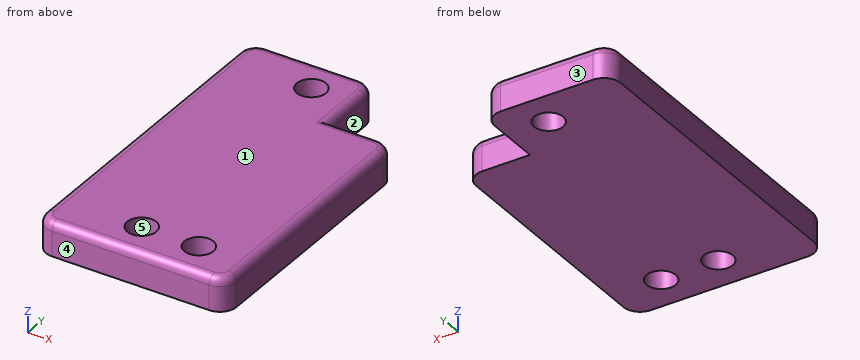
Autodesk Inventor part; units mm, degrees
ref_plane "Work Plane1" through (-7.86, -16.002, 12.7) normal (0, 0, 1) x (1, 0, 0)
ref_plane "YZ Plane" through (0, 0, 0) normal (1, 0, 0) x (0, 1, 0)
ref_plane "XZ Plane" through (0, 0, 0) normal (0, 1, 0) x (-1, 0, 0)
ref_plane "Work Plane1" through (-7.86, -16.002, 12.7) normal (0, 0, 1) x (1, 0, 0)
sketch "Sketch5" plane through (0, 0, 0) normal (0, 0, 1) x (1, 0, 0)
  line L0 (7.248, 20) -> (7.248, 11.68)
  line L1 (-5.86, 20) -> (7.248, 20)
  arc A0 (-5.86, 20) -> (-7.86, 18) centre (-5.86, 18) ccw
  line L2 (-7.86, 11.68) -> (-7.86, 18)
  line L3 (-3.792, 11.68) -> (-7.86, 11.68)
  line L4 (-3.792, 16.252) -> (-3.792, 11.68)
  line L5 (-0.752, 16.252) -> (-3.792, 16.252)
  line L6 (-0.752, 11.68) -> (-0.752, 16.252)
  line L7 (7.248, 11.68) -> (-0.752, 11.68)
  arc A1 (-7.86, -18) -> (-5.86, -20) centre (-5.86, -18) ccw
  line L8 (13, -20) -> (-5.86, -20)
  arc A2 (13, -20) -> (15, -18) centre (13, -18) ccw
  line L9 (15, -11.68) -> (15, -18)
  line L10 (-0.752, -11.68) -> (15, -11.68)
  line L11 (-0.752, -16.252) -> (-0.752, -11.68)
  line L12 (-3.792, -16.252) -> (-0.752, -16.252)
  line L13 (-3.792, -11.68) -> (-3.792, -16.252)
  line L14 (-7.86, -11.68) -> (-3.792, -11.68)
  line L15 (-7.86, -18) -> (-7.86, -11.68)
  line L16 (-0.752, 16.252) -> (-3.792, 16.252)
  line L17 (-3.792, 16.252) -> (-3.792, -16.252)
  line L18 (-3.792, -16.252) -> (-0.752, -16.252)
  line L19 (-0.752, -16.252) -> (-0.752, 16.252)
  line L20 (7.248, 11.68) -> (-7.86, 11.68)
  line L21 (-7.86, 11.68) -> (-7.86, -11.68)
  line L22 (-7.86, -11.68) -> (7.248, -11.68)
  line L23 (7.248, -11.68) -> (7.248, 11.68)
  line L24 (15, 11.43) -> (-1.002, 11.43)
  line L25 (15, 11.43) -> (7.248, 11.43)
  line L26 (7.248, 11.43) -> (7.248, -11.68)
  line L27 (7.248, -11.68) -> (15, -11.68)
  line L28 (15, -11.68) -> (15, 11.43)
  point P0 (0, 0)
extrude "Extrusion3" add sketch "Sketch5" along normal blind 4
sketch "Sketch6" plane through (0, 0, 4) normal (0, 0, 1) x (1, 0, 0)
  line L0 (7.248, 11.43) -> (7.248, 20)
  line L1 (7.248, 15.715) -> (2.248, 15.715)
  circle A0 centre (2.248, 15.715) radius 1.75
  line L2 (14.9228, 0) -> (0, 0)
  line L3 (7.248, 20) -> (7.248, 15.715)
  line L4 (15, -18) -> (15, 11.43)
  line L5 (15, -20) -> (15, -15.715)
  line L6 (15, -15.715) -> (-7.86, -15.715)
  line L7 (-7.86, 18) -> (-7.86, -18)
  line L8 (15, -15.715) -> (9, -15.715)
  circle A1 centre (9, -15.715) radius 1.75
  line L9 (-7.86, -15.715) -> (2.14, -15.715)
  circle A2 centre (2.14, -15.715) radius 1.75
  dimension "d14" = 5
  dimension "d15" = 3.5
  dimension "d16" = 4.285
  dimension "d17" = 6
  dimension "d18" = 3.5
  dimension "d19" = 10
  dimension "d20" = 3.5
extrude "Extrusion4" cut sketch "Sketch6" against normal blind 4
fillet "Fillet1" radius 2 2 edges at (7.248, 20, 2) (15, 11.43, 2)
fillet "Fillet2" radius 1 11 edges at (6.6622, 19.4142, 4) (-0.306, 20, 4) (-7.2742, 19.4142, 4) (-7.86, 0, 4) (-7.2742, -19.4142, 4) (3.57, -20, 4) (14.4142, -19.4142, 4) (15, -4.285, 4) (14.4142, 10.8442, 4) (10.124, 11.43, 4) (7.248, 14.715, 4)
properties part number "SyringeServoBaseClamp"
The listing builds one solid part. Answer for the finished solid, in the listing's coordinates (mm). Face numbers are marked on the shaded views. A direction names the side the tool comes from. Round coordinates to 2 decimals unless told otherwise and drop trailing zeros. Loops run counter-clockwise (first coordinate to the right, second up) from the corner with the lowest first, then second, coordinate; pieces in that order, holes last. Notation, with made-up numbers: M -38.75,64 L 10.25,64 A26 cw 10.25,83 Z; hole C 9,-39.75 d1. An arc over 180 degrees is marked long. Write each question's results on one line, items separated by ' | '. Start each with the question number.
1) Find section A-A on x = 9. Write down the section's boundary in (y, z) (3 decimals), plus the area to 3 significant figures.
2) Which of the six approach directions +Z, -Z, +X, -X, +Y, -Y give full straight-line access (tool end or side, diameter ignored) to the marked faces 1 and 2?
3) Find section C-C on z = 2.25. Write down the section's boundary in (x, y) (3 decimals).
4) Straight lines are drawn through the part: probe 1 along Y at (x, z) = (2.14, 1.4) (3 decimals); probe 2 along Y at (x, z) = (9, 2.6) (3 decimals); probe 3 along Y at (x, z) = (-6, 1.1). For each, find the intervals that lie inside material, in ascending order.
5) Find section B-B on x = 2.14. Write down the section's boundary in (y, z) (3 decimals), plus the area to 3 significant figures.
6) Find section D-D on y = 12.5. Write down the section's boundary in (x, z).
7) Determine the mould class of the marked faces 3, 4 and 5 for opening direction Y: pulls with the +Y half, pulls with the -Y half, needs draft (parallel to the pull), parting line crosses it, or undercut.
Final values:
1) outline: M -20,0 L -17.465,0 L -17.465,4 L -19,4 A1 ccw -20,3 Z; M -13.965,0 L 11.43,0 L 11.43,3 A1 ccw 10.43,4 L -13.965,4 Z | area: 111 mm²
2) face 1: +Z, +X, -X, +Y, -Y | face 2: +Z, -Z, +X, +Y
3) outline: M -7.86,-18 A2 ccw -5.86,-20 L 13,-20 A2 ccw 15,-18 L 15,9.43 A2 ccw 13,11.43 L 7.248,11.43 L 7.248,18 A2 ccw 5.248,20 L -5.86,20 A2 ccw -7.86,18 Z; hole C 2.14,-15.715 d3.5; hole C 2.248,15.715 d3.5; hole C 9,-15.715 d3.5
4) probe 1: -20 to -17.465, -13.965 to 13.968, 17.462 to 20 | probe 2: -20 to -17.465, -13.965 to 11.43 | probe 3: -20 to 20
5) outline: M -20,0 L -17.465,0 L -17.465,4 L -19,4 A1 ccw -20,3 Z; M -13.965,0 L 13.968,0 L 13.968,4 L -13.965,4 Z; M 17.462,0 L 20,0 L 20,3 A1 ccw 19,4 L 17.462,4 Z | area: 132 mm²
6) outline: M -7.86,0 L 7.25,0 L 7.25,3 A1 ccw 6.25,4 L -6.86,4 A1 ccw -7.86,3 Z
7) face 3: pulls with the +Y half | face 4: pulls with the -Y half | face 5: undercut
